```python
from build123d import *

# Parameters (mm, degrees)
BOSS_EXTRUDE1_DEPTH = 47.5
SKETCH2_R           = 1.5
CUT_EXTRUDE1_DEPTH  = 8
SKETCH3_R           = 11.2
BOSS_EXTRUDE2_DEPTH = 2
SKETCH4_R           = 2.5
BOSS_EXTRUDE3_DEPTH = 22.5
CUT_EXTRUDE2_START  = -8
SKETCH5_OUTSIDE_W   = 62.668
SKETCH5_OUTSIDE_H   = 62.668
CUT_EXTRUDE2_DEPTH  = 31.5


with BuildPart() as part:
    # Sketch1 → Boss-Extrude1 (new body)
    with BuildSketch(Plane(origin=(0, 0, 0), x_dir=(1, 0, 0), z_dir=(0, 1, 0))):
        with BuildLine():
            Line((-16.408001097, 21), (16.408001097, 21))
            ThreePointArc((16.408001097, 21), (18.844395719, 18.844395719), (21, 16.408001097))
            Line((21, 16.408001097), (21, -16.408001097))
            ThreePointArc((21, -16.408001097), (18.844395719, -18.844395719), (16.408001097, -21))
            Line((16.408001097, -21), (-16.408001097, -21))
            ThreePointArc((-16.408001097, -21), (-18.844395719, -18.844395719), (-21, -16.408001097))
            Line((-21, -16.408001097), (-21, 16.408001097))
            ThreePointArc((-21, 16.408001097), (-18.844395719, 18.844395719), (-16.408001097, 21))
        make_face()
    extrude(amount=BOSS_EXTRUDE1_DEPTH)

    # Sketch2 → Cut-Extrude1 (cut)
    with BuildSketch(Plane(origin=(0, 47.5, 0), x_dir=(1, 0, 0), z_dir=(0, 1, 0))):
        with Locations((-15.499780644, 15.499780644)):
            Circle(SKETCH2_R)
        with Locations((-15.499780644, -15.499780644)):
            Circle(SKETCH2_R)
        with Locations((15.499780644, -15.499780644)):
            Circle(SKETCH2_R)
        with Locations((15.499780644, 15.499780644)):
            Circle(SKETCH2_R)
    extrude(amount=-CUT_EXTRUDE1_DEPTH, mode=Mode.SUBTRACT)

    # Sketch3 → Boss-Extrude2 (add)
    with BuildSketch(Plane(origin=(0, 47.5, 0), x_dir=(1, 0, 0), z_dir=(0, 1, 0))):
        Circle(SKETCH3_R)
    extrude(amount=BOSS_EXTRUDE2_DEPTH)

    # Sketch4 → Boss-Extrude3 (add)
    with BuildSketch(Plane(origin=(0, 49.5, 0), x_dir=(1, 0, 0), z_dir=(0, 1, 0))):
        Circle(SKETCH4_R)
    extrude(amount=BOSS_EXTRUDE3_DEPTH)

    # Sketch5 outside → Cut-Extrude2 (cut)
    with BuildSketch(Plane(origin=(0, 47.5, 0), x_dir=(1, 0, 0), z_dir=(0, 1, 0)).offset(CUT_EXTRUDE2_START)):
        Rectangle(SKETCH5_OUTSIDE_W, SKETCH5_OUTSIDE_H)
        with BuildLine():
            Line((-20.5, 16.234916076), (-20.5, -16.234916076))
            ThreePointArc((-20.5, -16.234916076), (-18.490842328, -18.490842328), (-16.234916076, -20.5))
            Line((-16.234916076, -20.5), (16.234916076, -20.5))
            ThreePointArc((16.234916076, -20.5), (18.490842328, -18.490842328), (20.5, -16.234916076))
            Line((20.5, -16.234916076), (20.5, 16.234916076))
            ThreePointArc((20.5, 16.234916076), (18.490842328, 18.490842328), (16.234916076, 20.5))
            Line((16.234916076, 20.5), (-16.234916076, 20.5))
            ThreePointArc((-16.234916076, 20.5), (-18.490842328, 18.490842328), (-20.5, 16.234916076))
        make_face(mode=Mode.SUBTRACT)
    extrude(amount=-CUT_EXTRUDE2_DEPTH, mode=Mode.SUBTRACT)


solid = part.part
```
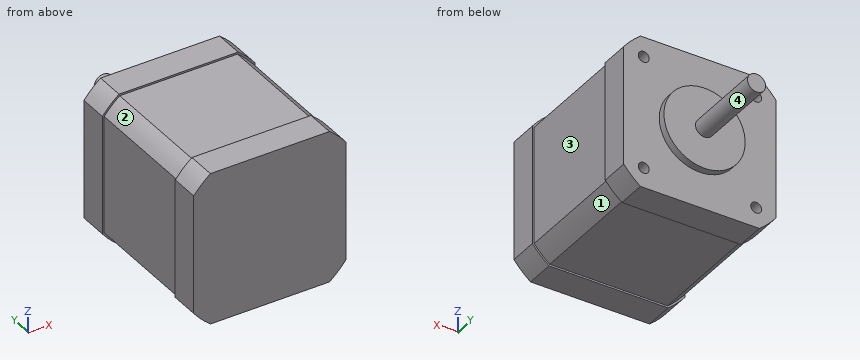
Part model, mm, in its own coordinate system. Face numbers are marked on the shaded views. A direction names the side the tool comes from. Round coordinates to 2 decimals unless told otherwise and drop trailing zeros. Order: outer loops, then holes, each group sorted by start corner. A loop starts at its lowest first (then second) coordinate and runs counter-clockwise, first axis right, second up. Notation, with made-up numbers: M 19.25,-27 L 54.25,-27 A32 cw 54.25,4 Z; hole C -19,59.25 d9. An arc over 180 degrees is marked long. Put each result on its own line as item: value. Start each with the question number.
1. Drop flat-ended pins along their axis: pin 1 (9.5 mm diameter, centred on x = 6, y = 29, fed in from +Z); pin 2 (1.5 mm diameter, centred on y = 16, z = -16, fed in from -X); pin 3 (1.5 mm diameter, centred on x = 15.5, z = 16, fed in from +Y). Give the stop position or say it passes through.
2. Slice it at C-C on z = 0. List the corners of the cut face in (x, y).
3. Drill centre lines: probe 1 along Z at (x, y) = (-13.5, 29); probe 2 along Y at (x, z) = (-3.5, -10.5); probe 3 along Y at (x, z) = (-12.5, 0.5). Where is each one in solid material? Low to high. Write a range as [from, to].
4. Slice it at B-B on y = 35.5. List the corners of the cut face in (x, z).
5. Slice it at D-D on x = 0. List the corners of the cut face in (y, z).
6. Slice it at A-A on x = 12.5. List the corners of the cut face in (y, z).
7. Tool access for the marked faces 1, 2, 3 and 4: list every direction of +Z, -Z, +X, -X, +Y, -Y with a clear straight run to the whole face (end or side of a thin tool).
Findings:
1. pin 1: z = 20.5
1. pin 2: x = -20.5
1. pin 3: y = 39.5
2. outline: M -21,0 L 21,0 L 21,8 L 20.5,8 L 20.5,39.5 L 21,39.5 L 21,47.5 L 11.2,47.5 L 11.2,49.5 L 2.5,49.5 L 2.5,72 L -2.5,72 L -2.5,49.5 L -11.2,49.5 L -11.2,47.5 L -21,47.5 L -21,39.5 L -20.5,39.5 L -20.5,8 L -21,8 Z
3. probe 1: [-20.5, 20.5]
3. probe 2: [0, 49.5]
3. probe 3: [0, 47.5]
4. outline: M -20.5,-16.23 A26.15 ccw -16.23,-20.5 L 16.23,-20.5 A26.15 ccw 20.5,-16.23 L 20.5,16.23 A26.15 ccw 16.23,20.5 L -16.23,20.5 A26.15 ccw -20.5,16.23 Z
5. outline: M 0,-21 L 8,-21 L 8,-20.5 L 39.5,-20.5 L 39.5,-21 L 47.5,-21 L 47.5,-11.2 L 49.5,-11.2 L 49.5,-2.5 L 72,-2.5 L 72,2.5 L 49.5,2.5 L 49.5,11.2 L 47.5,11.2 L 47.5,21 L 39.5,21 L 39.5,20.5 L 8,20.5 L 8,21 L 0,21 Z
6. outline: M 0,-21 L 8,-21 L 8,-20.5 L 39.5,-20.5 L 39.5,-21 L 47.5,-21 L 47.5,21 L 39.5,21 L 39.5,20.5 L 8,20.5 L 8,21 L 0,21 Z
7. face 1: -Z, +X
7. face 2: +Z, -X
7. face 3: +Z, -Z, +X
7. face 4: +Y
